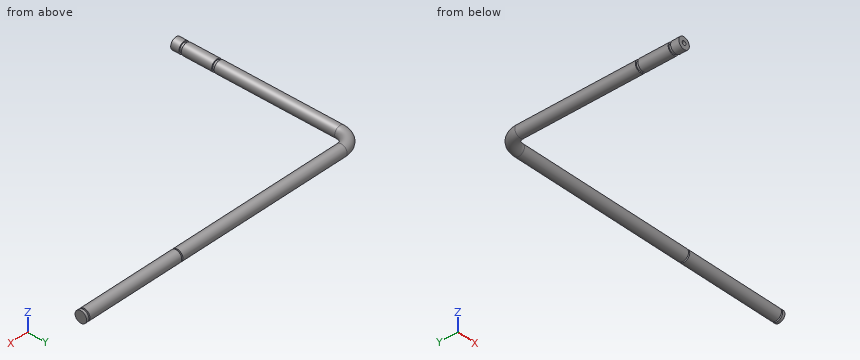
```python
from build123d import *

# Parameters (mm, degrees)
WYCI_GNI_CIE_PO_CIE_CE1_PROFILE_R = 3.5
SZKIC26_R                         = 4
SZKIC26_R_2                       = 2.85
WYTNIJ_WYCI_GNI_CIE1_DEPTH        = 1.5
SZKIC36_R                         = 4
SZKIC36_R_2                       = 2.85
WYTNIJ_WYCI_GNI_CIE3_DEPTH        = 1.5
SZKIC46_R                         = 4
SZKIC46_R_2                       = 1.6
WYTNIJ_WYCI_GNI_CIE4_DEPTH        = 0.8
WYTNIJ_WYCI_GNI_CIE5_START        = 0.8
SZKIC53_R                         = 4
SZKIC53_R_2                       = 1.6
WYTNIJ_WYCI_GNI_CIE5_DEPTH        = 0.8
SZKIC54_R                         = 1.25
WYTNIJ_WYCI_GNI_CIE6_DEPTH        = 10


with BuildPart() as part:
    # Wyciągnięcie po ścieżce1: sweep along a path in Szkic1
    with BuildLine(Plane.XY) as wyci_gni_cie_po_cie_ce1_path:
        Line((183, 0), (10, 0))
        ThreePointArc((10, 0), (2.928932188, -2.928932188), (0, -10))
        Line((0, -10), (0, -110))
    # Wyciągnięcie po ścieżce1 profile (on start of the path) → Wyciągnięcie po ścieżce1 (sweep)
    with BuildSketch(Plane(origin=(183, 0, 0), x_dir=(0, 0, -1), z_dir=(-1, 0, 0))):
        Circle(WYCI_GNI_CIE_PO_CIE_CE1_PROFILE_R)
    sweep(path=wyci_gni_cie_po_cie_ce1_path.line)

    # Szkic26 → Wytnij-wyciągnięcie1 (cut)
    with BuildSketch(Plane(origin=(0, -105, 0), x_dir=(-1, 0, 0), z_dir=(0, -1, 0))):
        Circle(SZKIC26_R)
        with Locations(Location((0, 0, 0), (0, 0, 180))):
            Circle(SZKIC26_R_2, mode=Mode.SUBTRACT)
    extrude(amount=-WYTNIJ_WYCI_GNI_CIE1_DEPTH, mode=Mode.SUBTRACT)

    # Szkic36 → Wytnij-wyciągnięcie3 (cut)
    with BuildSketch(Plane(origin=(0, -85, 0), x_dir=(-1, 0, 0), z_dir=(0, -1, 0))):
        Circle(SZKIC36_R)
        with Locations(Location((0, 0, 0), (0, 0, 180))):
            Circle(SZKIC36_R_2, mode=Mode.SUBTRACT)
    extrude(amount=-WYTNIJ_WYCI_GNI_CIE3_DEPTH, mode=Mode.SUBTRACT)

    # Szkic46 → Wytnij-wyciągnięcie4 (cut)
    with BuildSketch(Plane(origin=(181.5, 0, 0), x_dir=(0, 0, -1), z_dir=(1, 0, 0))):
        Circle(SZKIC46_R)
        with Locations(Location((0, 0, 0), (0, 0, 90))):
            Circle(SZKIC46_R_2, mode=Mode.SUBTRACT)
    extrude(amount=-WYTNIJ_WYCI_GNI_CIE4_DEPTH, mode=Mode.SUBTRACT)

    # Szkic53 → Wytnij-wyciągnięcie5 (cut)
    with BuildSketch(Plane(origin=(119, 0, 0), x_dir=(0, 0, -1), z_dir=(1, 0, 0)).offset(WYTNIJ_WYCI_GNI_CIE5_START)):
        Circle(SZKIC53_R)
        with Locations(Location((0, 0, 0), (0, 0, 90))):
            Circle(SZKIC53_R_2, mode=Mode.SUBTRACT)
    extrude(amount=-WYTNIJ_WYCI_GNI_CIE5_DEPTH, mode=Mode.SUBTRACT)

    # Szkic54 → Wytnij-wyciągnięcie6 (cut)
    with BuildSketch(Plane(origin=(0, -110, 0), x_dir=(-1, 0, 0), z_dir=(0, -1, 0))):
        with Locations(Location((0, 0, 0), (0, 0, 180))):
            Circle(SZKIC54_R)
    extrude(amount=-WYTNIJ_WYCI_GNI_CIE6_DEPTH, mode=Mode.SUBTRACT)


solid = part.part
```
Can you work these out from the model? Positions are in its coordinate system, mm. Coordinates: 2 decimals unless noted, no trailing zeros. Order: outer loops, then holes, each group sorted by start corner. A loop starts at its lowest first (then second) coordinate and runs counter-clockwise, first axis right, second up.
1. I'm going to push flat-ended pins straight in: pin 1 (2 mm diameter, centred on x = 0, z = 0, fed in from +Y); pin 2 (3.5 mm diameter, centred on x = -1, z = 0.5, fed in from +Y); pin 3 (2 mm diameter, centred on x = 1.5, z = 1, fed in from +Y). Where does each tip first touch, or does it pass through?
2. If we section it at A-A (x = 94.5): Please give me the cut outline in (y, z), then the cut area to 3 significant figures.
3. I need wall thicknesses on line 1 (X direction, y = -3, z = -0.75); line 2 (X direction, y = -54, z = 0.25); line 3 (Y direction, x = 153, z = -2). Which ranges of each line are inside material? Lowest first, please.
Entries:
1. pin 1: stops at y = 0.06
1. pin 2: stops at y = -0.2
1. pin 3: stops at y = 1.11
2. outline: circle Ø7 at (0, 0)
2. area: 38.5 mm2
3. line 1: x = -1.45 to 119, 119.8 to 180.7, 181.5 to 183
3. line 2: x = -3.49 to 3.49
3. line 3: y = -2.87 to 2.87
